Model file for the job. Use its own axes, mm. Round coordinates to 2 decimals unless told otherwise and drop trailing zeros. Write each loop counter-clockwise with the first axis right and the second up, starting at its lowest first coordinate (ties: lowest second). Pieces come first, ordered by that corner, then holes.
```python
from build123d import *

# Parameters (mm, degrees)
SKETCH1_W           = 200
SKETCH1_H           = 250
BOSS_EXTRUDE1_DEPTH = 6
SKETCH2_R           = 3.5
CUT_EXTRUDE1_DEPTH  = 6
FILLET1_R           = 10


with BuildPart() as part:
    # Sketch1 → Boss-Extrude1 (new body)
    with BuildSketch(Plane.XY):
        with Locations((100, 125)):
            Rectangle(SKETCH1_W, SKETCH1_H)
    extrude(amount=BOSS_EXTRUDE1_DEPTH)

    # Sketch2 → Cut-Extrude1 (cut)
    with BuildSketch(Plane(origin=(0, 0, 0), x_dir=(-1, 0, 0), z_dir=(0, 0, -1))):
        with Locations((-60, 65)):
            Circle(SKETCH2_R)
        with Locations((-85, 65)):
            Circle(SKETCH2_R)
        with Locations((-140, 65)):
            Circle(SKETCH2_R)
        with Locations((-115, 65)):
            Circle(SKETCH2_R)
        with Locations((-140, 185)):
            Circle(SKETCH2_R)
        with Locations((-115, 185)):
            Circle(SKETCH2_R)
        with Locations((-85, 185)):
            Circle(SKETCH2_R)
        with Locations((-60, 185)):
            Circle(SKETCH2_R)
    extrude(amount=-CUT_EXTRUDE1_DEPTH, mode=Mode.SUBTRACT)

    # Fillet1
    fillet1_edges = [part.edges().sort_by_distance(p)[0] for p in [
        (0, 250, 3),
        (200, 250, 3),
        (200, 0, 3),
        (0, 0, 3),
    ]]
    fillet(fillet1_edges, radius=FILLET1_R)


solid = part.part
```
1) Wall check: probe 1 along Y at (x, z) = (60, 4.7); probe 2 along X at (y, z) = (185, 1.8); probe 3 along Y at (x, z) = (88, 5). Give the ranges that are in metal, low to high.
2) Cut at B-B on y = 185. List the corners of the cut face in (x, z), and give its area (3 significant figures).
3) Pull direction Y, two halves, no side cores. Call faces 1 (the face through (200, 123, 3)), 2 (the face through (99, 250, 3)), 3 (the face through (81.767, 183.659, 2.958)): released by +Y, released by -Y, zero draft, split by the parting line, or undercut.
4) Cut at A-A on x = 140. List the corners of the cut face in (y, z).
Result sheet:
1. probe 1: y = 0 to 61.5, 68.5 to 181.5, 188.5 to 250
1. probe 2: x = 0 to 56.5, 63.5 to 81.5, 88.5 to 111.5, 118.5 to 136.5, 143.5 to 200
1. probe 3: y = 0 to 63.2, 66.8 to 183.2, 186.8 to 250
2. outline: (0, 0) - (56.5, 0) - (56.5, 6) - (0, 6) - close; (63.5, 0) - (81.5, 0) - (81.5, 6) - (63.5, 6) - close; (88.5, 0) - (111.5, 0) - (111.5, 6) - (88.5, 6) - close; (118.5, 0) - (136.5, 0) - (136.5, 6) - (118.5, 6) - close; (143.5, 0) - (200, 0) - (200, 6) - (143.5, 6) - close
2. area: 1,030 mm2
3. face 1: zero draft
3. face 2: released by +Y
3. face 3: undercut
4. outline: (0, 0) - (61.5, 0) - (61.5, 6) - (0, 6) - close; (68.5, 0) - (181.5, 0) - (181.5, 6) - (68.5, 6) - close; (188.5, 0) - (250, 0) - (250, 6) - (188.5, 6) - close
